Build history of the part. All positions in model axes, mm. Face numbers are marked on the shaded views. A direction names the side the tool comes from. Give positions to 0.01 mm unless a question says otherwise; leave off trailing zeros. Write each loop counter-clockwise with the first axis right and the second up, starting at its lowest first coordinate (ties: lowest second). Pieces come first, ordered by that corner, then holes. Notation, with made-up numbers: (55, 21) -> (81, 21) arc R23 cw to (81, 50) -> close; hole circle Ø5 at (74, 54). An arc over 180 degrees is marked (long way). Put each result on its own line as item: value.
from build123d import *

# Parameters (mm, degrees)
EXTRUDE_3_DEPTH     = 25
SKETCH_5_R          = 2.5
CUT_EXTRUDE_1_DEPTH = 35.528973341


with BuildPart() as part:
    # 草图3 → 凸台-拉伸3 (new, symmetric)
    with BuildSketch(Plane.XY):
        with BuildLine():
            Line((15, 1.5), (-15, 1.5))
            Line((-15, 1.5), (-15, 3))
            Line((-15, 3), (-3, 3))
            ThreePointArc((-3, 3), (-1.585786438, 3.585786438), (-1, 5))
            Line((-1, 5), (-1, 21.5))
            Line((-1, 21.5), (1, 21.5))
            Line((1, 21.5), (1, 5))
            ThreePointArc((1, 5), (1.585786438, 3.585786438), (3, 3))
            Line((3, 3), (15, 3))
            Line((15, 3), (15, 1.5))
        make_face()
    extrude(amount=EXTRUDE_3_DEPTH, both=True)

    # 草图5 → 切除-拉伸1 (cut, through all)
    with BuildSketch(Plane(origin=(0, 3, 0), x_dir=(1, 0, 0), z_dir=(0, 1, 0))):
        with Locations(Location((9, -10, 0), (0, 0, 270))):
            Circle(SKETCH_5_R)
    cut_extrude_1 = extrude(amount=-CUT_EXTRUDE_1_DEPTH, mode=Mode.SUBTRACT)

    # 镜向1: 切除-拉伸1 across plane
    add(cut_extrude_1.mirror(Plane(origin=(0, 0, 0), x_dir=(0, 0, 1), z_dir=(1, 0, 0))), mode=Mode.SUBTRACT)


solid = part.part
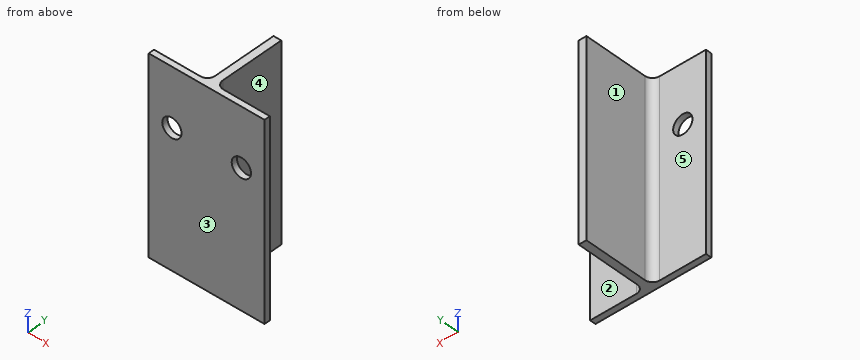
1) Slice it at B-B (x = -9). Write the cut outline in (y, z), plus the area to 3 significant figures.
Filled sheet:
outline: (1.5, -25) -> (3, -25) -> (3, 7.5) -> (1.5, 7.5) -> close; (1.5, 12.5) -> (3, 12.5) -> (3, 25) -> (1.5, 25) -> close
area: 67.5 mm2
2) Pull direction Y, two halves, no side cores. Call the marked faces 1, 2 and 3: released by +Y, released by -Y, zero draft, split by the parting line, or undercut.
Filled sheet:
face 1: zero draft
face 2: released by +Y
face 3: released by -Y
3) Wall check: L1, parallel to X at y = 2.35, z = 10; L2, parallel to Z at x = -9, y = 2.55; L3, parallel to X at y = 20.5, z = -19. Give the ranges that are in metal, low to high.
Filled sheet:
L1: -15 to -11.5, -6.5 to 6.5, 11.5 to 15
L2: -25 to 7.5, 12.5 to 25
L3: -1 to 1
4) Slice it at C-C (y = 14.5). Write the cut outline in (x, z), plus the area to 3 significant figures.
Filled sheet:
outline: (-1, -25) -> (1, -25) -> (1, 25) -> (-1, 25) -> close
area: 100 mm2
5) Slice it at D-D (x = 4.5). Write the cut outline in (y, z).
Filled sheet:
outline: (1.5, -25) -> (3, -25) -> (3, 25) -> (1.5, 25) -> close
6) Slice it at A-A (z = 10). Write the cut outline in (x, y).
Filled sheet:
outline: (-15, 1.5) -> (-11.5, 1.5) -> (-11.5, 3) -> (-15, 3) -> close; (-6.5, 1.5) -> (6.5, 1.5) -> (6.5, 3) -> (3, 3) arc R2 cw to (1, 5) -> (1, 21.5) -> (-1, 21.5) -> (-1, 5) arc R2 cw to (-3, 3) -> (-6.5, 3) -> close; (11.5, 1.5) -> (15, 1.5) -> (15, 3) -> (11.5, 3) -> close
7) Tool access for the marked faces 4 and 5: list every direction of +Z, -Z, +X, -X, +Y, -Y with a clear straight run to the whole face (end or side of a thin tool).
Filled sheet:
face 4: +Z, -Z, +X, +Y
face 5: +Z, -Z, -X, +Y
8) Pin check, flat tips, straight feed: pin 1 (12 mm diameter, centred on y = 13.5, z = -1.5, fed in from +X); pin 2 (3.5 mm diameter, centred on x = 11, z = 10.5, fed in from +Y); pin 3 (5 mm diameter, centred on y = 8, z = 7, fed in from -X). Stop position of each tip, or through.
Filled sheet:
pin 1: x = 1
pin 2: y = 3
pin 3: x = -1
